```python
from build123d import *

# Parameters (mm, degrees)
SKETCH13_R                                  = 2.5
RETANGULAR_PF20_12_PERFIL_2040_V_SLOT_DEPTH = 100


with BuildPart() as part:
    # Sketch13 → Retangular PF20-12 - PERFIL 2040 V-SLOT(1) (new body)
    with BuildSketch(Plane(origin=(0, 0, 0), x_dir=(-1, 0, 0), z_dir=(0, 1, 0))):
        with BuildLine():
            Line((-14.8, 10), (-13, 8.2))
            Line((-13, 8.2), (-15.5, 8.2))
            Line((-15.5, 8.2), (-15.5, 6.560660172))
            Line((-15.5, 6.560660172), (-12.939339828, 4))
            Line((-12.939339828, 4), (-10.3, 4))
            Line((-10.3, 4), (-10, 3.7))
            Line((-10, 3.7), (-9.7, 4))
            Line((-9.7, 4), (-7.060660172, 4))
            Line((-7.060660172, 4), (-4.5, 6.560660172))
            Line((-4.5, 6.560660172), (-4.5, 8.2))
            Line((-4.5, 8.2), (-7, 8.2))
            Line((-7, 8.2), (-5.2, 10))
            Line((-5.2, 10), (5.2, 10))
            Line((5.2, 10), (7, 8.2))
            Line((7, 8.2), (4.5, 8.2))
            Line((4.5, 8.2), (4.5, 6.560660172))
            Line((4.5, 6.560660172), (7.060660172, 4))
            Line((7.060660172, 4), (9.7, 4))
            Line((9.7, 4), (10, 3.7))
            Line((10, 3.7), (10.3, 4))
            Line((10.3, 4), (12.939339828, 4))
            Line((12.939339828, 4), (15.5, 6.560660172))
            Line((15.5, 6.560660172), (15.5, 8.2))
            Line((15.5, 8.2), (13, 8.2))
            Line((13, 8.2), (14.8, 10))
            Line((14.8, 10), (19, 10))
            ThreePointArc((19, 10), (19.707106781, 9.707106781), (20, 9))
            Line((20, 9), (20, 4.8))
            Line((20, 4.8), (18.2, 3))
            Line((18.2, 3), (18.2, 5.5))
            Line((18.2, 5.5), (16.560660172, 5.5))
            Line((16.560660172, 5.5), (14, 2.939339828))
            Line((14, 2.939339828), (14, 0.3))
            Line((14, 0.3), (13.7, 0))
            Line((13.7, 0), (14, -0.3))
            Line((14, -0.3), (14, -2.939339828))
            Line((14, -2.939339828), (16.560660172, -5.5))
            Line((16.560660172, -5.5), (18.2, -5.5))
            Line((18.2, -5.5), (18.2, -3))
            Line((18.2, -3), (20, -4.8))
            Line((20, -4.8), (20, -9))
            ThreePointArc((20, -9), (19.707106781, -9.707106781), (19, -10))
            Line((19, -10), (14.8, -10))
            Line((14.8, -10), (13, -8.2))
            Line((13, -8.2), (15.5, -8.2))
            Line((15.5, -8.2), (15.5, -6.560660172))
            Line((15.5, -6.560660172), (12.939339828, -4))
            Line((12.939339828, -4), (10.3, -4))
            Line((10.3, -4), (10, -3.7))
            Line((10, -3.7), (9.7, -4))
            Line((9.7, -4), (7.060660172, -4))
            Line((7.060660172, -4), (4.5, -6.560660172))
            Line((4.5, -6.560660172), (4.5, -8.2))
            Line((4.5, -8.2), (7, -8.2))
            Line((7, -8.2), (5.2, -10))
            Line((5.2, -10), (-5.2, -10))
            Line((-5.2, -10), (-7, -8.2))
            Line((-7, -8.2), (-4.5, -8.2))
            Line((-4.5, -8.2), (-4.5, -6.560660172))
            Line((-4.5, -6.560660172), (-7.060660172, -4))
            Line((-7.060660172, -4), (-9.7, -4))
            Line((-9.7, -4), (-10, -3.7))
            Line((-10, -3.7), (-10.3, -4))
            Line((-10.3, -4), (-12.939339828, -4))
            Line((-12.939339828, -4), (-15.5, -6.560660172))
            Line((-15.5, -6.560660172), (-15.5, -8.2))
            Line((-15.5, -8.2), (-13, -8.2))
            Line((-13, -8.2), (-14.8, -10))
            Line((-14.8, -10), (-19, -10))
            ThreePointArc((-19, -10), (-19.707106781, -9.707106781), (-20, -9))
            Line((-20, -9), (-20, -4.8))
            Line((-20, -4.8), (-18.2, -3))
            Line((-18.2, -3), (-18.2, -5.5))
            Line((-18.2, -5.5), (-16.560660172, -5.5))
            Line((-16.560660172, -5.5), (-14, -2.939339828))
            Line((-14, -2.939339828), (-14, -0.3))
            Line((-14, -0.3), (-13.7, 0))
            Line((-13.7, 0), (-14, 0.3))
            Line((-14, 0.3), (-14, 2.939339828))
            Line((-14, 2.939339828), (-16.560660172, 5.5))
            Line((-16.560660172, 5.5), (-18.2, 5.5))
            Line((-18.2, 5.5), (-18.2, 3))
            Line((-18.2, 3), (-20, 4.8))
            Line((-20, 4.8), (-20, 9))
            ThreePointArc((-20, 9), (-19.707106781, 9.707106781), (-19, 10))
            Line((-19, 10), (-14.8, 10))
        make_face()
        with Locations((-10, 0)):
            Circle(SKETCH13_R, mode=Mode.SUBTRACT)
        with Locations((10, 0)):
            Circle(SKETCH13_R, mode=Mode.SUBTRACT)
        Polygon((-2.7, 8.2), (-2.7, 6.239339828), (-6, 2.939339828), (-6, -2.939339828), (-2.7, -6.239339828), (-2.7, -8.2), (2.7, -8.2), (2.7, -6.239339828), (6, -2.939339828), (6, 2.939339828), (2.7, 6.239339828), (2.7, 8.2), align=None, mode=Mode.SUBTRACT)
    extrude(amount=RETANGULAR_PF20_12_PERFIL_2040_V_SLOT_DEPTH)


solid = part.part
```
Work out the finished part from the listing and answer in its coordinate system (mm). A direction names the side the tool comes from. Give positions to 0.01 mm unless a question says otherwise; leave off trailing zeros. Loops run counter-clockwise (first coordinate to the right, second up) from the corner with the lowest first, then second, coordinate; pieces in that order, holes last. Notation, with made-up numbers: (2, 5.5) -> (36, 5.5) arc R18 cw to (36, 29.5) -> close; hole circle Ø8 at (65.5, 2). An arc over 180 degrees is marked (long way). Write item = value, one per line. Start each with the question number.
(1) The mould has two halves that part along X. Classify faces 1 (the flat face through (20, 49, -7)), 2 (the flat face through (-5, 100, 5)), 3 (the flat face through (15.26, 49.3, 4.2)): +X half, -X half, draft (parallel to the pull), parting line (faces both ways), or undercut.
(2) Find section C-C on y = 94. Give the number of separate pieces and of enclosed holes in the cut face, and give its area (3 significant figures).
(3) Which of the six approach directions +Z, -Z, +X, -X, +Y, -Y give full straight-line access (tool end or side, diameter ignored) to faces 4 (the flat face through (14, 49, 2)), 5 (the flat face through (-12, 49, 4)), 6 (the flat face through (13.9, 49.3, -9.1)), 7 (the flat face through (-18.2, 49, 4))?
(4) Find section B-B on z = 1.25. Give the vertices of the cut face in (x, y), and give its area (3 significant figures).
(5) Given pin 1 Ø3 at (x, z) = (-13, -2) entering from -Y; pin 2 Ø1.3 at (y, z) = (69.5, -1.5) entering from -X; pin 3 Ø1.3 at (x, y) = (-11, 50) entering from +Z; pin 4 Ø2 at (x, y) = (9, 43) entering from -Z, each flat-ended and moving along its own axis, determine where each tip first touches the part or whether it passes through.
(6) Find the intervals of material crossed by probe 1 along Z at (x, y) = (10, 39.5); probe 2 along Z at (x, y) = (-9, 93); probe 3 along X at (y, z) = (33, -0.5), in increasing order. Write a range as from..to.
(7) Find section A-A on x = 0.5. Give the vertices of the cut face in (y, z), and give its area (3 significant figures).
From the geometry:
q1.face_1 = +X half
q1.face_2 = draft
q1.face_3 = undercut
q2.separate_pieces = 1
q2.enclosed_holes = 3
q2.area = 288 mm^2
q3.face_4 = +X, +Y, -Y
q3.face_5 = +Z, +Y, -Y
q3.face_6 = -Z, +Y, -Y
q3.face_7 = +Y, -Y
q4.outline = (-14, 0) -> (-12.17, 0) -> (-12.17, 100) -> (-14, 100) -> close; (-7.83, 0) -> (-6, 0) -> (-6, 100) -> (-7.83, 100) -> close; (6, 0) -> (7.83, 0) -> (7.83, 100) -> (6, 100) -> close; (12.17, 0) -> (14, 0) -> (14, 100) -> (12.17, 100) -> close
q4.area = 734 mm^2
q5.pin_1 = 0
q5.pin_2 = -14
q5.pin_3 = 4
q5.pin_4 = -4
q6.probe_1 = -3.7..-2.5, 2.5..3.7
q6.probe_2 = -4..-2.29, 2.29..4
q6.probe_3 = -14..-12.45, -7.55..-6, 6..7.55, 12.45..14
q7.outline = (0, -10) -> (100, -10) -> (100, -8.2) -> (0, -8.2) -> close; (0, 8.2) -> (100, 8.2) -> (100, 10) -> (0, 10) -> close
q7.area = 360 mm^2
